from build123d import *

# Parameters (mm, degrees)
SKETCH1_R           = 25.4
BOSS_EXTRUDE1_DEPTH = 80


with BuildPart() as part:
    # Sketch1 → Boss-Extrude1 (new body)
    with BuildSketch(Plane(origin=(0, 0, 0), x_dir=(1, 0, 0), z_dir=(0, 1, 0))):
        with Locations(Location((0, 0, 0), (0, 0, 270))):
            Circle(SKETCH1_R)
        Polygon((12.990381057, 7.5), (0, 15), (-12.990381057, 7.5), (-12.990381057, -7.5), (0, -15), (12.990381057, -7.5), align=None, mode=Mode.SUBTRACT)
    extrude(amount=-BOSS_EXTRUDE1_DEPTH)


solid = part.part
Design review of the part built by this model. Coordinates are the model's own, in mm. A direction names the side the tool comes from. Round coordinates to 2 decimals unless told otherwise and drop trailing zeros. Loops run counter-clockwise (first coordinate to the right, second up) from the corner with the lowest first, then second, coordinate; pieces in that order, holes last. Notation, with made-up numbers: (-12.5, 19) - (21.5, 19) arc R12 ccw to (21.5, 41) - close; hole circle Ø10 at (63, 56.25). An arc over 180 degrees is marked (long way). One line per question, with ' | ' between items.
1. We need section C-C, the plane x = -9. State the section outline as (y, z) points.
Results are:
outline: (-80, -23.75) - (0, -23.75) - (0, -9.8) - (-80, -9.8) - close; (-80, 9.8) - (0, 9.8) - (0, 23.75) - (-80, 23.75) - close
2. Draft analysis for pull direction Z (two halves, no side actions). For faces 3 (the face through (6.586, -39.44, -11.198)), 4 (the face through (6, 0, -12)), 5 (the face through (-15.456, -39.44, -20.157)), state which applies: released by +Z, released by -Z, zero draft, split by the parting line, or undercut.
Results are:
face 3: undercut | face 4: zero draft | face 5: split by the parting line
3. Clearance check with flat-ended pins moving along their axes: P1, Ø12, axis at y = -39, z = -1.5, coming from the +X side; P2, Ø4, axis at x = -6.5, y = -30, coming from the -Z side; P3, Ø4, axis at x = 15.5, y = -60.5, coming from the -Z side. State where each tip first meets the part, or that it passes through.
Results are:
P1: stops at x = 25.4 | P2: stops at z = -25 | P3: stops at z = -21.52
4. We need section A-A, the plane y = -42. State the section outline as (x, z) points.
Results are:
outline: circle Ø50.8 at (0, 0); hole (-12.99, -7.5) - (0, -15) - (12.99, -7.5) - (12.99, 7.5) - (0, 15) - (-12.99, 7.5) - close
5. We need section B-B, the plane z = 0. State the section outline as (x, y) points.
Results are:
outline: (-25.4, -80) - (-12.99, -80) - (-12.99, 0) - (-25.4, 0) - close; (12.99, -80) - (25.4, -80) - (25.4, 0) - (12.99, 0) - close
6. For L1, parallel to Z at x = -5.5, y = -48.5; L2, parallel to X at y = -22, z = 5.5; L3, parallel to X at y = -60.5, z = 13, list the stretches that pass through material, from the lowest coordinate up. Write a range as [from, to].
Results are:
L1: z = [-24.8, -11.82], [11.82, 24.8] | L2: x = [-24.8, -12.99], [12.99, 24.8] | L3: x = [-21.82, -3.46], [3.46, 21.82]
7. We need section D-D, the plane z = -20.5. State the section outline as (x, y) points.
Results are:
outline: (-15, -80) - (15, -80) - (15, 0) - (-15, 0) - close
8. For faces 1 (the face through (6, -80, -12)), 2 (the face through (-6.586, -39.44, 11.198)), list the 3-axis set-ups (+Z, -Z, +X, -X, +Y, -Y) from which the entire face can be reached by the end or side of a thin tool; tool diameter is ignored.
Results are:
face 1: +Z, -Z, +X, -X, -Y | face 2: +Y, -Y
